Input: dimensioned drawing with shaded views. Units: mm. Origin: part minimum x, y, z. Give positions to 0.01 mm unless a question says otherwise; leave off trailing zeros. Order: outer loops, then holes, each group sorted by start corner. A loop starts at its lowest first (then second) coordinate and runs counter-clockwise, first axis right, second up. Notation, with made-up numbers: (-25.5, 9.25) - (-11.5, 9.25) arc R16 cw to (-11.5, 20.25) - close; hole circle Ø2 at (71, 3.5). An arc over 180 degrees is marked (long way). Use a Markdown table: item, result.
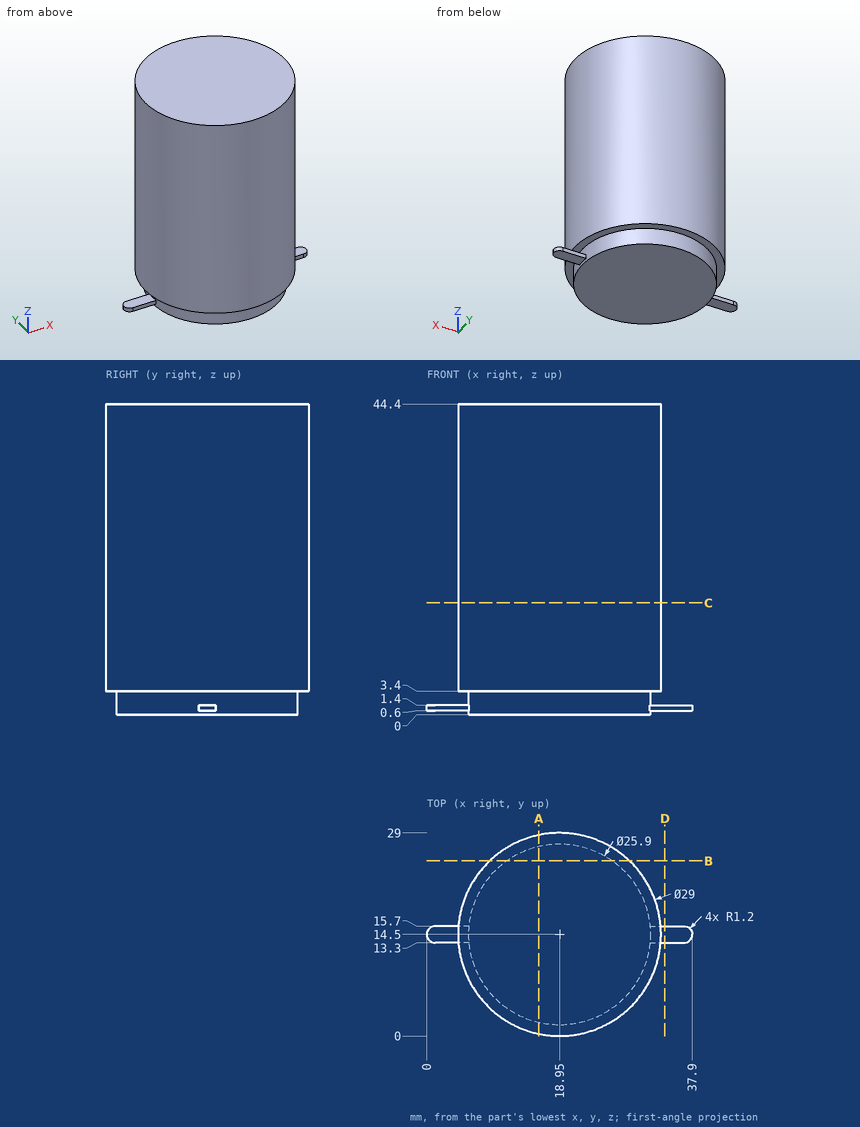
1. Material intervals for line 1 along Z through (x, y) = (6.5, 20.5); line 2 along X through (y, z) = (4, 8); line 3 along X through (y, z) = (25.25, 4), sorted ascending.
Response:
| item | result |
|---|---|
| line 1 | z = 3.4 to 44.4 |
| line 2 | x = 8.95 to 28.95 |
| line 3 | x = 9.22 to 28.68 |
2. Pin query (flat end, axial travel): pin 1 (0.6 mm diameter, centred on x = 3, z = 1, fed in from -Y); pin 2 (4 mm diameter, centred on x = 27.5, z = 18, fed in from -Y); pin 3 (0.7 mm diameter, centred on x = 3.5, y = 15, fed in from -Z); pin 4 (8.5 mm diameter, centred on x = 19.5, y = 16.5, fed in from -Z). Return the tip coordinate at first contact, or that it passes through.
Response:
| item | result |
|---|---|
| pin 1 | stops at y = 13.3 |
| pin 2 | stops at y = 1.56 |
| pin 3 | stops at z = 0.6 |
| pin 4 | stops at z = 0 |
3. Section query B-B (y = 25). Return loops of the section in (x, z).
Response:
| item | result |
|---|---|
| outline | (8.95, 3.4) - (11.37, 3.4) - (11.37, 0) - (26.53, 0) - (26.53, 3.4) - (28.95, 3.4) - (28.95, 44.4) - (8.95, 44.4) - close |
4. Section query A-A (x = 16). Return loops of the section in (y, z).
Response:
| item | result |
|---|---|
| outline | (0.3, 3.4) - (1.89, 3.4) - (1.89, 0) - (27.11, 0) - (27.11, 3.4) - (28.7, 3.4) - (28.7, 44.4) - (0.3, 44.4) - close |
5. Section query D-D (x = 34). Return loops of the section in (y, z), then the cut area to 3 significant figures.
Response:
| item | result |
|---|---|
| outline | (13.3, 0.6) - (15.7, 0.6) - (15.7, 1.4) - (13.3, 1.4) - close |
| area | 1.92 mm^2 |
6. Section query C-C (z = 16). Return loops of the section in (x, y).
Response:
| item | result |
|---|---|
| outline | circle Ø29 at (18.95, 14.5) |
